Design review of the part built by this model. Coordinates are the model's own, in mm. A direction names the side the tool comes from. Round coordinates to 2 decimals unless told otherwise and drop trailing zeros. Order: outer loops, then holes, each group sorted by start corner. A loop starts at its lowest first (then second) coordinate and runs counter-clockwise, first axis right, second up. Notation, with made-up numbers: (89, -35.75) - (147, -35.75) arc R24 cw to (147, 1.25) - close; hole circle Ø9 at (15.25, 23). An arc over 180 degrees is marked (long way). Write item = value, one per line.
from build123d import *

# Parameters (mm, degrees)
SKETCH_1_R          = 8
SKETCH_1_W          = 8.2
SKETCH_1_H          = 8.2
EXTRUDE_1_DEPTH     = 5
SKETCH_2_W          = 8.2
SKETCH_2_H          = 5
EXTRUDE_2_DEPTH     = 27
SKETCH_3_W          = 8.2
SKETCH_3_H          = 5
EXTRUDE_3_DEPTH     = 27
SKETCH_4_R          = 7
SKETCH_4_W          = 8.2
SKETCH_4_H          = 8.2
EXTRUDE_4_DEPTH     = 4
CUT_EXTRUDE_1_DEPTH = 6
FILLET_1_R          = 2
FILLET_2_R          = 2


with BuildPart() as part:
    # 草图1 → 凸台-拉伸1 (new body)
    with BuildSketch(Plane.XY):
        Circle(SKETCH_1_R)
        Rectangle(SKETCH_1_W, SKETCH_1_H, mode=Mode.SUBTRACT)
    extrude(amount=EXTRUDE_1_DEPTH)

    # 草图2 → 凸台-拉伸2 (add)
    with BuildSketch(Plane.XZ.offset(-4.1)):
        with Locations((0, 2.5)):
            Rectangle(SKETCH_2_W, SKETCH_2_H)
    extrude(amount=-EXTRUDE_2_DEPTH)

    # 草图3 → 凸台-拉伸3 (add)
    with BuildSketch(Plane(origin=(0, -4.1, 0), x_dir=(1, 0, 0), z_dir=(0, 1, 0))):
        with Locations((0, -2.5)):
            Rectangle(SKETCH_3_W, SKETCH_3_H)
    extrude(amount=-EXTRUDE_3_DEPTH)

    # 草图4 → 凸台-拉伸4 (add)
    with BuildSketch(Plane.XY.offset(5)):
        Circle(SKETCH_4_R)
        Rectangle(SKETCH_4_W, SKETCH_4_H, mode=Mode.SUBTRACT)
    extrude(amount=EXTRUDE_4_DEPTH)

    # 草图5 → 切除-拉伸1 (cut, through all)
    with BuildSketch(Plane.XY.offset(5)):
        with BuildLine():
            Line((2.15, 27.5), (2.15, 9.5))
            ThreePointArc((2.15, 9.5), (0, 7.35), (-2.15, 9.5))
            Line((-2.15, 9.5), (-2.15, 27.5))
            ThreePointArc((-2.15, 27.5), (0, 29.65), (2.15, 27.5))
        make_face()
    cut_extrude_1 = extrude(amount=-CUT_EXTRUDE_1_DEPTH, mode=Mode.SUBTRACT)

    # 镜向1: 切除-拉伸1 across plane
    add(cut_extrude_1.mirror(Plane.ZX), mode=Mode.SUBTRACT)

    # 圆角1
    fillet_1_edges = [part.edges().sort_by_distance(p)[0] for p in [
        (-4.1, 6.869497798, 2.5),
        (4.1, 6.869497798, 2.5),
        (4.1, -6.869497798, 2.5),
        (-4.1, -6.869497798, 2.5),
    ]]
    fillet(fillet_1_edges, radius=FILLET_1_R)

    # 圆角2
    fillet_2_edges = [part.edges().sort_by_distance(p)[0] for p in [
        (-4.1, 31.1, 2.5),
        (4.1, 31.1, 2.5),
        (4.1, -31.1, 2.5),
        (-4.1, -31.1, 2.5),
    ]]
    fillet(fillet_2_edges, radius=FILLET_2_R)


solid = part.part
1) We need section B-B on y = -12. Write out the cut boundary in (x, z).
Findings:
outline = (-4.1, 0) - (-2.15, 0) - (-2.15, 5) - (-4.1, 5) - close; (2.15, 0) - (4.1, 0) - (4.1, 5) - (2.15, 5) - close
2) We need section A-A on z = 3.5. Write out the cut boundary in (x, y).
Findings:
outline = (-4.88, -6.34) arc R2 cw to (-4.1, -7.92) - (-4.1, -29.1) arc R2 ccw to (-2.1, -31.1) - (2.1, -31.1) arc R2 ccw to (4.1, -29.1) - (4.1, -7.92) arc R2 cw to (4.88, -6.34) arc R8 ccw to (4.88, 6.34) arc R2 cw to (4.1, 7.92) - (4.1, 29.1) arc R2 ccw to (2.1, 31.1) - (-2.1, 31.1) arc R2 ccw to (-4.1, 29.1) - (-4.1, 7.92) arc R2 cw to (-4.88, 6.34) arc R8 ccw to start; hole (-4.1, -4.1) - (4.1, -4.1) - (4.1, 4.1) - (-4.1, 4.1) - close; hole (-2.15, -27.5) arc R2.15 ccw to (2.15, -27.5) - (2.15, -9.5) arc R2.15 ccw to (-2.15, -9.5) - close; hole (-2.15, 9.5) arc R2.15 ccw to (2.15, 9.5) - (2.15, 27.5) arc R2.15 ccw to (-2.15, 27.5) - close
3) To check wall thickness, follow L1, parallel to Y at x = 2.25, z = 4.75; L2, parallel to X at y = 1, z = 1; L3, parallel to X at y = -23, z = 4.75. State the ranges of each line that lie inside material, in increasing order. Write a range as from..to.
Findings:
L1 = -31.09..-4.1, 4.1..31.09
L2 = -7.94..-4.1, 4.1..7.94
L3 = -4.1..-2.15, 2.15..4.1
4) We need section C-C on x = -3. Write out the cut boundary in (y, z).
Findings:
outline = (-30.89, 0) - (-4.1, 0) - (-4.1, 9) - (-6.32, 9) - (-6.32, 5) - (-30.89, 5) - close; (4.1, 0) - (30.89, 0) - (30.89, 5) - (6.32, 5) - (6.32, 9) - (4.1, 9) - close
5) The part is to be moulded in two halves that separate along Y. For faces 1 (the cylindrical face through (-3.53, 30.5, 2.54)), 2 (the flat face through (2.15, 19, 3)), 3 (the cylindrical face through (-8, 0, 2)), say which applies: released by +Y, released by -Y, zero draft, split by the parting line, or undercut.
Findings:
face_1 = released by +Y
face_2 = undercut
face_3 = split by the parting line
6) Clearance check with flat-ended pins moving along their axes: pin 1 Ø2.5 at (y, z) = (-16.5, 1.5) entering from -X; pin 2 Ø2.5 at (y, z) = (1.5, 5) entering from -X; pin 3 Ø2.5 at (y, z) = (-21.5, 3.5) entering from +X. State where each tip first meets the part, or that it passes through.
Findings:
pin_1 = -4.1
pin_2 = -8
pin_3 = 4.1
7) We need section D-D on z = 6.5. Write out the cut boundary in (x, y), and give its area (3 significant figures).
Findings:
outline = circle Ø14 at (0, 0); hole (-4.1, -4.1) - (4.1, -4.1) - (4.1, 4.1) - (-4.1, 4.1) - close
area = 86.7 mm^2
8) For faces 4 (the flat face through (4.1, 0, 4)), 5 (the flat face through (-4.1, -18, 3)), 6 (the flat face through (4.1, 18, 2)), list the 3-axis set-ups (+Z, -Z, +X, -X, +Y, -Y) from which the entire face can be reached by the end or side of a thin tool; tool diameter is ignored.
Findings:
face_4 = +Z, -Z
face_5 = +Z, -Z, -X, -Y
face_6 = +Z, -Z, +X, +Y
